Part model, mm, in its own coordinate system. A direction names the side the tool comes from. Give positions to 0.01 mm unless a question says otherwise; leave off trailing zeros. Order: outer loops, then holes, each group sorted by start corner. A loop starts at its lowest first (then second) coordinate and runs counter-clockwise, first axis right, second up. Notation, with made-up numbers: (1, 88) - (5, 88) arc R22 cw to (5, 98) - close; hole circle Ø11 at (-15, 58). An arc over 180 degrees is marked (long way). One line per item, written item: value.
```python
from build123d import *

# Parameters (mm, degrees)
BOSS_EXTRUDE1_DEPTH = 9.6
SKETCH2_R           = 2.1
CUT_EXTRUDE1_DEPTH  = 20.628805364
SKETCH3_R           = 3.65
BOSS_EXTRUDE5_DEPTH = 5
SKETCH3_4_R         = 2.45
CUT_EXTRUDE4_DEPTH  = 5
CUT_EXTRUDE5_DEPTH  = 0.6
CUT_EXTRUDE6_DEPTH  = 2.2
CUT_EXTRUDE7_DEPTH  = 2
CUT_EXTRUDE8_START  = -4
CUT_EXTRUDE8_DEPTH  = 4
CHAMFER1_SIZE       = 0.6
CUT_EXTRUDE9_DEPTH  = 20.498782013


with BuildPart() as part:
    # Sketch1 → Boss-Extrude1 (new body)
    with BuildSketch(Plane(origin=(0, 0, 0), x_dir=(1, 0, 0), z_dir=(0, 1, 0))):
        with BuildLine():
            ThreePointArc((13.5, 3.3), (16.8, 0), (13.5, -3.3))
            Line((13.5, -3.3), (-13.5, -3.3))
            ThreePointArc((-13.5, -3.3), (-16.8, 0), (-13.5, 3.3))
            Line((-13.5, 3.3), (13.5, 3.3))
        make_face()
    extrude(amount=BOSS_EXTRUDE1_DEPTH)

    # Sketch2 → Cut-Extrude1 (cut, through all)
    with BuildSketch(Plane(origin=(0, 9.6, 0), x_dir=(1, 0, 0), z_dir=(0, 1, 0))):
        with Locations(Location((-13.5, 0, 0), (0, 0, 270))):
            Circle(SKETCH2_R)
    cut_extrude1 = extrude(amount=-CUT_EXTRUDE1_DEPTH, mode=Mode.SUBTRACT)

    # Mirror1: Cut-Extrude1 across plane
    add(cut_extrude1.mirror(Plane(origin=(0, 0, 0), x_dir=(0, 0, 1), z_dir=(1, 0, 0))), mode=Mode.SUBTRACT)

    # Sketch3 → Boss-Extrude5 (add, symmetric)
    with BuildSketch(Plane(origin=(0, 4.8, 0), x_dir=(1, 0, 0), z_dir=(0, 1, 0))):
        with Locations(Location((3.8, 0, 0), (0, 0, 270))):
            Circle(SKETCH3_R)
    extrude(amount=BOSS_EXTRUDE5_DEPTH, both=True)

    # Sketch3<4> → Cut-Extrude4 (cut, symmetric)
    with BuildSketch(Plane(origin=(0, 4.8, 0), x_dir=(1, 0, 0), z_dir=(0, 1, 0))):
        with Locations(Location((3.8, 0, 0), (0, 0, 270))):
            Circle(SKETCH3_4_R)
    extrude(amount=CUT_EXTRUDE4_DEPTH, both=True, mode=Mode.SUBTRACT)

    # Sketch6 → Cut-Extrude5 (cut)
    with BuildSketch(Plane(origin=(0, 9.6, 0), x_dir=(1, 0, 0), z_dir=(0, 1, 0))):
        with BuildLine():
            Line((-4.6, 3.3), (-4.6, -3.3))
            Line((-4.6, -3.3), (2.240352604, -3.3))
            ThreePointArc((2.240352604, -3.3), (0.15, 0), (2.240352604, 3.3))
            Line((2.240352604, 3.3), (-4.6, 3.3))
        make_face()
    cut_extrude5 = extrude(amount=-CUT_EXTRUDE5_DEPTH, mode=Mode.SUBTRACT)

    # Mirror2: Cut-Extrude5 across plane
    add(cut_extrude5.mirror(Plane.ZX.offset(4.8)), mode=Mode.SUBTRACT)

    # Sketch8 → Cut-Extrude6 (cut)
    with BuildSketch(Plane.XZ):
        with BuildLine():
            Line((13.5, 3.3), (5.359647396, 3.3))
            ThreePointArc((5.359647396, 3.3), (7.45, 0), (5.359647396, -3.3))
            Line((5.359647396, -3.3), (13.5, -3.3))
            ThreePointArc((13.5, -3.3), (16.8, 0), (13.5, 3.3))
        make_face()
    cut_extrude6 = extrude(amount=-CUT_EXTRUDE6_DEPTH, mode=Mode.SUBTRACT)

    # Mirror3: Cut-Extrude6 across plane
    add(cut_extrude6.mirror(Plane.ZX.offset(4.8)), mode=Mode.SUBTRACT)

    # Sketch9 → Cut-Extrude7 (cut)
    with BuildSketch(Plane(origin=(0, 7.4, 0), x_dir=(1, 0, 0), z_dir=(0, 1, 0))):
        with BuildLine():
            Line((6.785381048, 2.1), (10.954415588, 2.1))
            ThreePointArc((10.954415588, 2.1), (10.289796635, 0), (10.954415588, -2.1))
            Line((10.954415588, -2.1), (6.785381048, -2.1))
            ThreePointArc((6.785381048, -2.1), (7.45, 0), (6.785381048, 2.1))
        make_face()
    cut_extrude7 = extrude(amount=-CUT_EXTRUDE7_DEPTH, mode=Mode.SUBTRACT)

    # Mirror4: Cut-Extrude7 across plane
    add(cut_extrude7.mirror(Plane.ZX.offset(4.8)), mode=Mode.SUBTRACT)

    # Sketch11 → Cut-Extrude8 (cut)
    with BuildSketch(Plane(origin=(0, 9.6, 0), x_dir=(1, 0, 0), z_dir=(0, 1, 0)).offset(CUT_EXTRUDE8_START)):
        with BuildLine():
            Line((-10.954415588, 2.1), (-4.6, 2.1))
            Line((-4.6, 2.1), (-4.6, -2.1))
            Line((-4.6, -2.1), (-10.954415588, -2.1))
            ThreePointArc((-10.954415588, -2.1), (-10.2, 0), (-10.954415588, 2.1))
        make_face()
    cut_extrude8 = extrude(amount=CUT_EXTRUDE8_DEPTH, mode=Mode.SUBTRACT)

    # Mirror7: Cut-Extrude8 across plane
    add(cut_extrude8.mirror(Plane.ZX.offset(4.8)), mode=Mode.SUBTRACT)

    # Chamfer1
    chamfer1_edges = [part.edges().sort_by_distance(p)[0] for p in [
        (-4.6, 9.6, 2.7),
        (-4.6, 9.6, -2.7),
        (-4.6, 0, -2.7),
        (-4.6, 0, 2.7),
    ]]
    chamfer(chamfer1_edges, length=CHAMFER1_SIZE - 0.0001)  # a hair under: the kernel refuses the full size

    # Sketch13 → Cut-Extrude9 (cut, through all)
    with BuildSketch(Plane(origin=(0, 9, 0), x_dir=(1, 0, 0), z_dir=(0, 1, 0))):
        with BuildLine():
            Line((0.814618952, -2.1), (-3.4, -2.1))
            Line((-3.4, -2.1), (-3.4, 2.1))
            Line((-3.4, 2.1), (0.814618952, 2.1))
            ThreePointArc((0.814618952, 2.1), (0.15, 0), (0.814618952, -2.1))
        make_face()
    extrude(amount=-CUT_EXTRUDE9_DEPTH, mode=Mode.SUBTRACT)


solid = part.part
```
1) Drill centre lines: line 1 along X through (y, z) = (8.5, 0); line 2 along Z through (x, y) = (-6.5, 1.5); line 3 along X through (y, z) = (7.5, 1.25). Where is each one in solid material? Low to high. Write a range as from..to.
Outcome:
line 1: x = -16.8..-15.6, -11.4..-10.2, -4.6..-3.4, 0.15..1.35, 6.25..7.45
line 2: z = -3.3..-2.1, 2.1..3.3
line 3: x = -16.55..-15.19, -11.81..-10.45, -4.6..-3.4, 0.37..1.69, 5.91..7.23
2) Pin check, flat tips, straight feed: pin 1 (3 mm diameter, centred on x = -6, y = 2.5, fed in from +Z); pin 2 (3 mm diameter, centred on x = 12, z = 1.5, fed in from +Y); pin 3 (2 mm diameter, centred on x = -2, z = -1, fed in from +Y); pin 4 (2 mm diameter, centred on x = -10.5, z = 1.5, fed in from +Y). Stop position of each tip, or through.
Outcome:
pin 1: stops at z = 3.3
pin 2: stops at y = 7.4
pin 3: passes through
pin 4: stops at y = 9.6
3) Cut at C-C, the plane y = 4.5. Give the cut face in (x, z), then the cut area to 3 significant figures.
Outcome:
outline: (-13.5, -3.3) - (2.24, -3.3) arc R3.65 ccw to (5.36, -3.3) - (13.5, -3.3) arc R3.3 ccw to (13.5, 3.3) - (5.36, 3.3) arc R3.65 ccw to (2.24, 3.3) - (-13.5, 3.3) arc R3.3 ccw to start; hole circle Ø4.2 at (-13.5, 0); hole (-3.4, -2.1) - (0.81, -2.1) arc R3.65 cw to (0.81, 2.1) - (-3.4, 2.1) - close; hole circle Ø4.9 at (3.8, 0); hole circle Ø4.2 at (13.5, 0)
area: 152 mm^2
4) Cut at A-A, the plane x = 3.8. Give the cut face in (y, z).
Outcome:
outline: (-0.2, -3.65) - (9.8, -3.65) - (9.8, -2.45) - (-0.2, -2.45) - close; (-0.2, 2.45) - (9.8, 2.45) - (9.8, 3.65) - (-0.2, 3.65) - close
5) Mould opens along Z. For faces 1 (the flat face through (1, -0.2, 1)), 2 (the cylindrical face through (16.8, 4.8, -0.1)), 3 (the flat face through (-8, 8, -2.1)) say: released by +Z, released by -Z, zero draft, split by the parting line, or undercut.
Outcome:
face 1: zero draft
face 2: split by the parting line
face 3: undercut
6) Cut at D-D, the plane x = 10. Give the cut face in (y, z).
Outcome:
outline: (2.2, -3.3) - (7.4, -3.3) - (7.4, -2.1) - (5.4, -2.1) - (5.4, 2.1) - (7.4, 2.1) - (7.4, 3.3) - (2.2, 3.3) - (2.2, 2.1) - (4.2, 2.1) - (4.2, -2.1) - (2.2, -2.1) - close
7) Cut at B-B, the plane y = 7. Give the cut face in (x, z).
Outcome:
outline: (-13.5, -3.3) - (2.24, -3.3) arc R3.65 ccw to (5.36, -3.3) - (13.5, -3.3) arc R3.3 ccw to (13.5, 3.3) - (5.36, 3.3) arc R3.65 ccw to (2.24, 3.3) - (-13.5, 3.3) arc R3.3 ccw to start; hole circle Ø4.2 at (-13.5, 0); hole (-10.95, -2.1) - (-4.6, -2.1) - (-4.6, 2.1) - (-10.95, 2.1) arc R3.3 cw to start; hole (-3.4, -2.1) - (0.81, -2.1) arc R3.65 cw to (0.81, 2.1) - (-3.4, 2.1) - close; hole circle Ø4.9 at (3.8, 0); hole (6.79, -2.1) - (10.95, -2.1) arc R3.65 cw to (10.95, 2.1) - (6.79, 2.1) arc R3.65 cw to start; hole circle Ø4.2 at (13.5, 0)
8) Which spindle directions (+Z, -Z, +X, -X, +Y, -Y) get a long thin tool onto all of the face, cutting with end or side? Do faces 4 (the flat face through (-1, 5, 2.1)), 5 (the flat face through (-11, 0, 0)), 6 (the flat face through (-8, 5.6, 0)), 7 (the flat face through (-4.6, 2, 0)). Say none if no direction does.
Outcome:
face 4: +Y, -Y
face 5: +Z, -Z, -X, -Y
face 6: +Y
face 7: -Y
